Geometry check sheet. Reference: the model listing, model coordinates, mm. A direction names the side the tool comes from. Round coordinates to 2 decimals unless told otherwise and drop trailing zeros. Order: outer loops, then holes, each group sorted by start corner. A loop starts at its lowest first (then second) coordinate and runs counter-clockwise, first axis right, second up.
(1) Release check for a two-part mould opening along Z. For faces 3 (the face through (-0.54, -2.44, 7.89)), 4 (the face through (-1.193, 9.087, 21.423)), 5 (the face through (0, 0, 16)), 6 (the face through (-2.5, 9, 16)) record: +Z half, -Z half, draft (parallel to the pull), parting line (faces both ways), or undercut.
(2) Sectioned sample at A-A (y = 0). Record the boundary of the cut face in (x, z) (3 decimals), plus the area to 3 significant figures.
(3) Sectioned sample at D-D (z = 18.25). Record the boundary of the cut face in (x, y) (3 decimals).
(4) Sectioned sample at C-C (z = 11.75). Record the boundary of the cut face in (x, y), plus the area to 3 significant figures.
(5) Material ranges on line 1 along Y through (x, z) = (0, 5); line 2 along Z through (x, y) = (8.5, 5.75); line 3 along X through (y, z) = (-1, 15.25), recorded low to high.
(6) Go/stop test with flat-tipped pins: pin 1 (6 mm diameter, centred on x = 4, z = 15, fed in from -Y); pin 2 (1 mm diameter, centred on y = -6, z = 13.5, fed in from +X); pin 3 (4 mm diameter, centred on x = -0.5, z = 19, fed in from -Y) (3 decimals). Record where each tip stops, or that it passes through.
(7) Set-up check for faces 1 (the face through (-2.5, 9, 27)), 2 (the face through (0, 0, 28)): record each of +Z, -Z, +X, -X, +Y, -Y from which the full face is reachable in a straight line by a thin tool's end or side.
from build123d import *

# Parameters (mm, degrees)
SKETCH_1_R      = 11
SKETCH_1_R_2    = 2.5
EXTRUDE_1_DEPTH = 16
SKETCH_2_R      = 9.165
EXTRUDE_2_DEPTH = 11
SKETCH_3_R      = 11
EXTRUDE_3_DEPTH = 1


with BuildPart() as part:
    # 草图1 → 凸台-拉伸1 (new body)
    with BuildSketch(Plane.XY):
        Circle(SKETCH_1_R)
        Circle(SKETCH_1_R_2, mode=Mode.SUBTRACT)
    extrude(amount=EXTRUDE_1_DEPTH)

    # 草图2 → 凸台-拉伸2 (add)
    with BuildSketch(Plane.XY.offset(16)):
        Circle(SKETCH_2_R)
    extrude(amount=EXTRUDE_2_DEPTH)

    # 草图3 → 凸台-拉伸3 (add)
    with BuildSketch(Plane.XY.offset(27)):
        Circle(SKETCH_3_R)
    extrude(amount=EXTRUDE_3_DEPTH)


solid = part.part
Answer below:
1. face 3: draft
1. face 4: undercut
1. face 5: -Z half
1. face 6: undercut
2. outline: (-11, 0) - (-2.5, 0) - (-2.5, 16) - (2.5, 16) - (2.5, 0) - (11, 0) - (11, 16) - (9.165, 16) - (9.165, 27) - (11, 27) - (11, 28) - (-11, 28) - (-11, 27) - (-9.165, 27) - (-9.165, 16) - (-11, 16) - close
2. area: 496 mm2
3. outline: circle Ø18.33 at (0, 0)
4. outline: circle Ø22 at (0, 0); hole circle Ø5 at (0, 0)
4. area: 360 mm2
5. line 1: y = -11 to -2.5, 2.5 to 11
5. line 2: z = 0 to 16, 27 to 28
5. line 3: x = -10.95 to -2.29, 2.29 to 10.95
6. pin 1: stops at y = -10.95
6. pin 2: stops at x = 9.53
6. pin 3: stops at y = -9.165
7. face 1: none
7. face 2: +Z, +X, -X, +Y, -Y
